from build123d import *


with BuildPart() as part:
    # Sketch1 → Revolve1 (revolve)
    with BuildSketch(Plane.XY):
        Polygon((25.4, 1.5875), (14.400348017, 1.499999985), (12.900348032, 0), (0, 0), (0, 3.175), (50.8, 3.175), (50.8, 0), (37.899651968, 0), (36.4, 1.5875), align=None)
    revolve(axis=Axis((0, 3.175, 0), (1, 0, 0)))

    # Sketch6 → M3 Clearance Hole1 (revolve, cut)
    with BuildSketch(Plane.ZX.offset(3.175)):
        Polygon((0, 0), (0, 7.371463052), (1.7, 6.35), (1.7, 0), align=None)
    m3_clearance_hole1 = revolve(axis=Axis((-6.35, 3.175, 0), (1, 0, 0)), mode=Mode.SUBTRACT)

    # Mirror1: M3 Clearance Hole1 across plane
    add(m3_clearance_hole1.mirror(Plane.ZY.offset(-25.4)), mode=Mode.SUBTRACT)


solid = part.part
Input: part model. Units: mm. Frame: model coordinates. A direction names the side the tool comes from. Give positions to 0.01 mm unless a question says otherwise; leave off trailing zeros. Loops run counter-clockwise (first coordinate to the right, second up) from the corner with the lowest first, then second, coordinate; pieces in that order, holes last. Notation, with made-up numbers: M 66.5,-24 L 72.5,-24 A23 ccw 72.5,-6 Z; hole C 70,30.5 d7. An arc over 180 degrees is marked long. Use CSV: the item, a comma, the result in double quotes.
(1) Pin query (flat end, axial travel): P1, Ø2, axis at y = 3, z = 0.5, coming from the -X side; P2, Ø3, axis at x = 39, z = -2, coming from the -Y side; P3, Ø2, axis at y = 3.175, z = 0, coming from the -X side. Return the tip coordinate at first contact, or that it passes through.
Outcome:
P1,"stops at x = 6.45"
P2,"stops at y = 0.04"
P3,"stops at x = 6.77"
(2) Section A-A, the plane x = 5.5. Return loops of the section in (y, z) (3 decimals), plus the area to 3 significant figures.
Outcome:
outline,"C 3.175,0 d6.35; hole C 3.175,0 d3.4"
area,"22.6 mm²"
(3) Pull-direction query (Y, two-part tool) for faces 4 (the face through (50.8, 5, 1)), 5 (the face through (30.82, 1.66, -0.48)), 6 (the face through (7.19, 3.44, 0.14)); classes: pulls with the +Y half, pulls with the -Y half, needs draft (parallel to the pull), parting line crosses it, or undercut.
Outcome:
face 4,"needs draft"
face 5,"parting line crosses it"
face 6,"undercut"
(4) Set-up query: faces 1 (the face through (47.669, 4.835, -0.369)), 2 (the face through (19.823, 4.805, -0.072)), 3 (the face through (3.131, 4.835, -0.369)). Return all of +Z, -Z, +X, -X, +Y, -Y with unobstructed straight access to the full face (end or side cutting, diameter ignored); none if empty.
Outcome:
face 1,"+X"
face 2,"none"
face 3,"-X"
(5) Material intervals for L1, parallel to Y at x = 47, z = 0 (3 decimals); L2, parallel to Y at x = 9, z = -0.25; L3, parallel to Y at x = 3, z = 1.5 (3 decimals), sorted ascending. Write a range as [from, to].
Outcome:
L1,"y = [0, 1.475], [4.875, 6.35]"
L2,"y = [0.01, 6.34]"
L3,"y = [0.377, 2.375], [3.975, 5.973]"
(6) Section B-B, the plane x = 27. Return loops of the section in (y, z) (1 decimal), plus the area to 3 significant figures.
Outcome:
outline,"C 3.2,0 d3.2"
area,"7.92 mm²"
